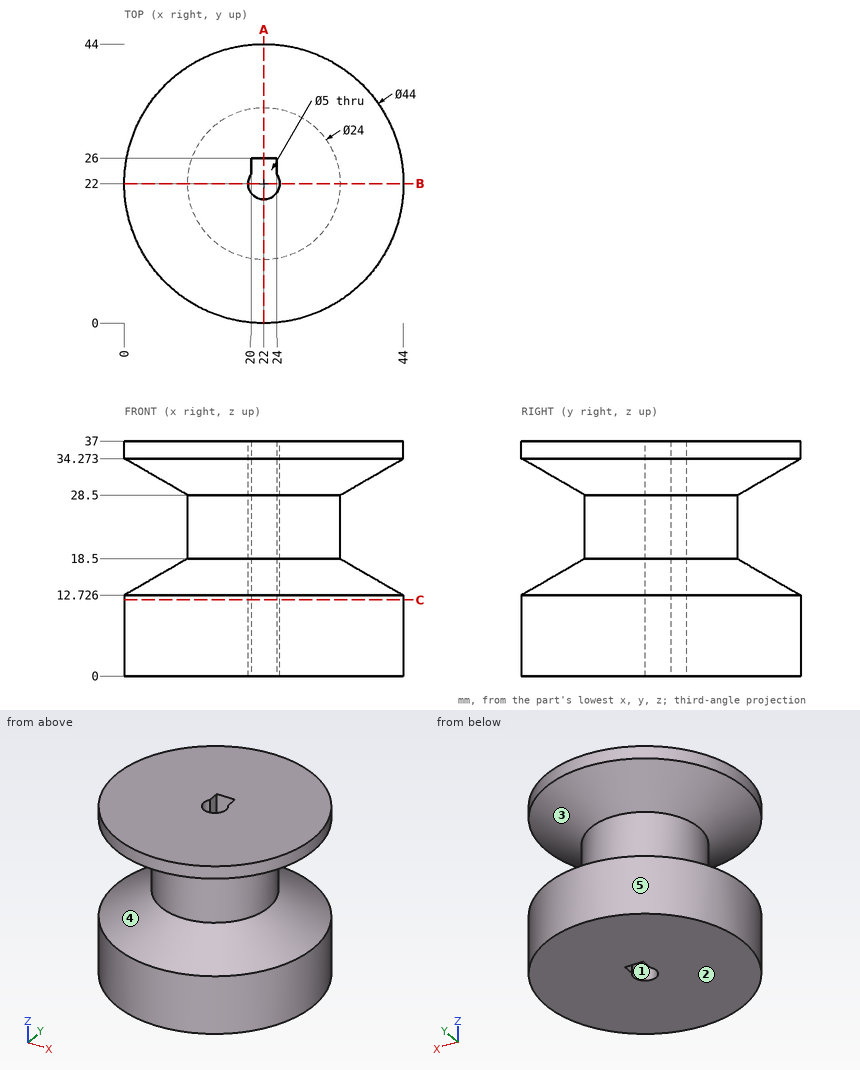
Verification items for this drawing (mm, ordinates from the low corner). A direction names the side the tool comes from. Give positions to 0.01 mm unless a question says otherwise; leave off trailing zeros. Loops run counter-clockwise (first coordinate to the right, second up) from the corner with the lowest first, then second, coordinate; pieces in that order, holes last. Notation, with made-up numbers: M 79,69.25 L 133,69.25 A17 ccw 133,78.25 Z; hole C 46.5,-24.75 d9. An arc over 180 degrees is marked long. Answer in a Markdown table with one row per item.
1) Thickness scan on line 1 (X direction, y = 22, z = 11); line 2 (Z direction, x = 6.5, y = 8.5); line 3 (Z direction, x = 29, y = 32). Record the ranges inside material, lowest first.
Solutions:
| item | result |
|---|---|
| line 1 | x = 0 to 19.5, 24.5 to 44 |
| line 2 | z = 0 to 13.56, 33.44 to 37 |
| line 3 | z = 0 to 18.38, 28.62 to 37 |
2) Cross-section at C-C (z = 12). Enter the section's corners in (x, y).
Solutions:
| item | result |
|---|---|
| outline | C 22,22 d44; hole M 20,23.5 A2.5 ccw long 24,23.5 L 24,26 L 20,26 Z |
3) Cross-section at A-A (x = 22). Enter the section's corners in (y, z), plus the area to 3 significant figures.
Solutions:
| item | result |
|---|---|
| outline | M 0,0 L 19.5,0 L 19.5,37 L 0,37 L 0,34.27 L 10,28.5 L 10,18.5 L 0,12.73 Z; M 26,0 L 44,0 L 44,12.73 L 34,18.5 L 34,28.5 L 44,34.27 L 44,37 L 26,37 Z |
| area | 1,070 mm^2 |
4) Cross-section at B-B (y = 22). Enter the section's corners in (x, z).
Solutions:
| item | result |
|---|---|
| outline | M 0,0 L 19.5,0 L 19.5,37 L 0,37 L 0,34.27 L 10,28.5 L 10,18.5 L 0,12.73 Z; M 24.5,0 L 44,0 L 44,12.73 L 34,18.5 L 34,28.5 L 44,34.27 L 44,37 L 24.5,37 Z |
5) Depth check by flat-ended pin: pin 1 (2 mm diameter, centred on y = 25, z = 20.5, fed in from -X); pin 2 (10 mm diameter, centred on x = 21, z = 26.5, fed in from -Y); pin 3 (3 mm diameter, centred on y = 33, z = 25, fed in from -X); pin 4 (12 mm diameter, centred on x = 12.5, y = 23.5, fed in from -Z). Enter the tip coordinate at first touch or a pass-through.
Solutions:
| item | result |
|---|---|
| pin 1 | stops at x = 10.17 |
| pin 2 | stops at y = 4.83 |
| pin 3 | stops at x = 14.67 |
| pin 4 | stops at z = 0 |
6) Tool access check on the marked faces 4 and 5. Record the directions out of +Z, -Z, +X, -X, +Y, -Y that give a thin tool (end or side, any length) a straight path to the whole face; none if there is none.
Solutions:
| item | result |
|---|---|
| face 4 | none |
| face 5 | +Z, -Z |
7) Mould release check, pull along Z, two halves, no side actions. Record for the marked faces 1, 2 and 3: released by +Z, released by -Z, zero draft, split by the parting line, or undercut.
Solutions:
| item | result |
|---|---|
| face 1 | zero draft |
| face 2 | released by -Z |
| face 3 | undercut |
